Geometry check sheet. Reference: the model listing, model coordinates, mm. A direction names the side the tool comes from. Round coordinates to 2 decimals unless told otherwise and drop trailing zeros. Write each loop counter-clockwise with the first axis right and the second up, starting at its lowest first coordinate (ties: lowest second). Pieces come first, ordered by that corner, then holes. Notation, with made-up numbers: (11.5, 17) -> (47.5, 17) arc R22 ccw to (47.5, 50) -> close; hole circle Ø9 at (89.25, 39.5). An arc over 180 degrees is marked (long way). Put each result on its own line as item: value. Start each with the question number.
Solid Edge part; units mm, degrees
sketch "Sketch1" plane through (0, 0, 0) normal (0, -1, 0) x (1, 0, 0)
  line L0 (0, 30) -> (0, 0)
  line L1 (0, 0) -> (2.5, 0)
  line L2 (2.5, 28) -> (2.5, 0)
  line L3 (1.25, 28) -> (2.5, 28)
  line L4 (1.25, 29) -> (1.25, 28)
  line L5 (2.5, 29) -> (1.25, 29)
  line L6 (2.5, 30) -> (2.5, 29)
  line L7 (2.5, 30) -> (0, 30)
extrude "Protrusion1" add sketch "Sketch1" against normal blind 80
sketch "Sketch2" plane through (0, 0, 0) normal (0, -1, 0) x (1, 0, 0)
  line L0 (1.75, -2.5) -> (1.75, 0)
  line L1 (1, 0) -> (1.75, 0)
  line L2 (1, 0) -> (1, -3)
  line L3 (1, -3) -> (2.5, -3)
  line L4 (2.5, -3) -> (2.5, -2.5)
  line L5 (2.5, -2.5) -> (1.75, -2.5)
extrude "Vysunutí_2" add sketch "Sketch2" against normal blind 80
sketch "Sketch3" plane through (1.25, 40, 30) normal (0, 0, 1) x (0, 1, 0)
  line L0 (-37, 0) -> (-38, 0)
  line L1 (-38, 0) -> (-38, -1.25)
  line L2 (-38, -1.25) -> (-37, -1.25)
  line L3 (-37, -1.25) -> (-37, 0)
extrude "Cutout1" cut sketch "Sketch3" against normal blind 30
sketch "Sketch4" plane through (0, 40, 15) normal (-1, 0, 0) x (0, -1, 0)
  line L0 (-20, 5) -> (-20, 1)
  line L1 (-20, 1) -> (-30, 1)
  line L2 (-30, 1) -> (-30, 5)
  line L3 (-30, 5) -> (-20, 5)
  line L4 (15, 5) -> (15, 1)
  line L5 (15, 1) -> (20, 1)
  line L6 (25, 1) -> (20, 1)
  line L7 (25, 5) -> (25, 1)
  line L8 (20, 5) -> (25, 5)
  line L9 (20, 5) -> (15, 5)
extrude "Protrusion2" add sketch "Sketch4" along normal blind 5
sketch "Sketch5" plane through (-2.5, 20, 16) normal (0, 0, -1) x (1, 0, 0)
  line L0 (-2.5, -5) -> (-2.5, 5)
  line L1 (-2.5, 5) -> (-0.5, 5)
  line L2 (-0.5, 5) -> (-0.5, -5)
  line L3 (-0.5, -5) -> (-2.5, -5)
  line L4 (-0.5, -50) -> (-0.5, -40)
  line L5 (-0.5, -40) -> (-2.5, -40)
  line L6 (-2.5, -40) -> (-2.5, -50)
  line L7 (-2.5, -50) -> (-0.5, -50)
extrude "Vysunutí_4" add sketch "Sketch5" along normal blind 10
(1) Mould release check, pull along X, two halves, no side actions. Record for faces 1 (the flat face through (-4, 60, 15)), 2 (the flat face through (-1, 65, 16)), 3 (the flat face through (2.5, 41, 14)): +X half, -X half, draft (parallel to the pull), parting line (faces both ways), or undercut.
(2) Sectioned sample at A-A (x = -1.5). Record the cut outline in (y, z), and give its area (3 significant figures).
(3) Sectioned sample at C-C (y = 8.5). Record the cut outline in (x, z), and give its area (3 significant figures).
(4) Material ranges on L1, parallel to Y at x = 1.75, z = 17; L2, parallel to Y at x = -4.5, z = 18; L3, parallel to Z at x = 1.5, y = 56, recorded low to high. Write a range as from..to.
(5) Sectioned sample at D-D (z = 23.5). Record the cut outline in (x, y).
(6) Sectioned sample at B-B (z = 15). Record the cut outline in (x, y).
(7) Go/stop test with flat-tipped pins: pin 1 Ø2.5 at (x, y) = (-1.5, 21) entering from -Z; pin 2 Ø1.5 at (x, y) = (-3, 61) entering from +Z; pin 3 Ø2 at (x, y) = (-4.5, 64) entering from -Z. Record where each tip stops, or that it passes through.
(8) Set-up check for faces 4 (the flat face through (-1, 20, 16)), 5 (the flat face through (1.75, 39, -1)), 6 (the flat face through (-4, 25, 15)): record each of +Z, -Z, +X, -X, +Y, -Y from which the full face is reachable in a straight line by a thin tool's end or side.
Found:
1. face 1: draft
1. face 2: undercut
1. face 3: +X half
2. outline: (15, 16) -> (25, 16) -> (25, 20) -> (15, 20) -> close; (60, 16) -> (70, 16) -> (70, 20) -> (60, 20) -> close
2. area: 80.0 mm2
3. outline: (0, 0) -> (1, 0) -> (1, -3) -> (2.5, -3) -> (2.5, -2.5) -> (1.75, -2.5) -> (1.75, 0) -> (2.5, 0) -> (2.5, 28) -> (1.25, 28) -> (1.25, 29) -> (2.5, 29) -> (2.5, 30) -> (0, 30) -> close
3. area: 76.4 mm2
4. L1: 0..2, 3..80
4. L2: 15..25, 60..70
4. L3: -3..28, 29..30
5. outline: (0, 0) -> (2.5, 0) -> (2.5, 2) -> (1.25, 2) -> (1.25, 3) -> (2.5, 3) -> (2.5, 80) -> (0, 80) -> close
6. outline: (-5, 15) -> (-3, 15) -> (-3, 25) -> (-5, 25) -> close; (-5, 60) -> (-3, 60) -> (-3, 70) -> (-5, 70) -> close; (0, 0) -> (2.5, 0) -> (2.5, 2) -> (1.25, 2) -> (1.25, 3) -> (2.5, 3) -> (2.5, 80) -> (0, 80) -> close
7. pin 1: z = 16
7. pin 2: z = 20
7. pin 3: z = 6
8. face 4: -Z, +Y, -Y
8. face 5: +X, +Y, -Y
8. face 6: +Z, -Z, -X
